Check sheet for the modelled part. Datum: model origin and axes. Units: mm. A direction names the side the tool comes from. Give positions to 0.01 mm unless a question says otherwise; leave off trailing zeros. Order: outer loops, then holes, each group sorted by start corner. A loop starts at its lowest first (then second) coordinate and runs counter-clockwise, first axis right, second up.
from build123d import *

# Parameters (mm, degrees)
F1_DEPTH  = 15
F3_DEPTH  = 2.6
F5_DEPTH  = 2.6
F6_R      = 2.5
F7_DEPTH  = 15.001
F9_DEPTH  = 25
F10_W     = 7.263658
F10_H     = 12.422406
F11_DEPTH = 25.43
F13_DEPTH = 13.301


with BuildPart() as f1:
    # F0 (on Top) → F1 (new body)
    with BuildSketch(Plane.XY):
        with BuildLine():
            Line((0, 10.7), (0, 0))
            Line((0, 0), (16.8, 0))
            Line((16.8, 0), (16.8, -2.6))
            Line((16.8, -2.6), (68.5, -2.6))
            Line((68.5, -2.6), (68.5, 3.1))
            Line((68.5, 3.1), (57, 3.1))
            ThreePointArc((57, 3.1), (54.75, 5.35), (57, 7.6))
            Line((57, 7.6), (68.5, 7.6))
            Line((68.5, 7.6), (68.5, 13.3))
            Line((68.5, 13.3), (16.8, 13.3))
            Line((16.8, 13.3), (16.8, 10.7))
            Line((16.8, 10.7), (0, 10.7))
        make_face()
        with BuildLine():
            Line((50.53, 0.57), (50.53, -1.1))
            Line((50.53, -1.1), (47.93, -1.1))
            Line((47.93, -1.1), (47.93, 0.37))
            Line((47.93, 0.37), (42.93, 0.37))
            Line((42.93, 0.37), (42.93, -1.1))
            Line((42.93, -1.1), (36.03, -1.1))
            Line((36.03, -1.1), (36.03, 11.8))
            Line((36.03, 11.8), (42.93, 11.8))
            Line((42.93, 11.8), (42.93, 10.33))
            Line((42.93, 10.33), (47.93, 10.33))
            Line((47.93, 10.33), (47.93, 11.8))
            Line((47.93, 11.8), (50.53, 11.8))
            Line((50.53, 11.8), (50.53, 10.13))
            ThreePointArc((50.53, 10.13), (45.75, 5.35), (50.53, 0.57))
        make_face(mode=Mode.SUBTRACT)
        with BuildLine():
            Line((25.897848, 2.656896), (25.897848, 0.656896))
            Line((25.897848, 0.656896), (24.897848, 0.656896))
            Line((24.897848, 0.656896), (23.134171, 1.6))
            Line((23.134171, 1.6), (10.6, 1.6))
            Line((10.6, 1.6), (10.6, 9.1))
            Line((10.6, 9.1), (23.134171, 9.1))
            Line((23.134171, 9.1), (24.897848, 10.043104))
            Line((24.897848, 10.043104), (25.897848, 10.043104))
            Line((25.897848, 10.043104), (25.897848, 8.043104))
            ThreePointArc((25.897848, 8.043104), (24.4, 5.35), (25.897848, 2.656896))
        make_face(mode=Mode.SUBTRACT)
    extrude(amount=F1_DEPTH)

    # F2 (on face) → F3 (cut, through all)
    with BuildSketch(Plane.XZ.offset(2.6)):
        Polygon((16.8, 15), (16.8, 0), (25.530007, 15), align=None)
    extrude(amount=-F3_DEPTH, mode=Mode.SUBTRACT)

    # F4 (on face) → F5 (cut, through all)
    with BuildSketch(Plane(origin=(0, 13.3, 0), x_dir=(-1, 0, 0), z_dir=(0, 1, 0))):
        Polygon((-25.53, 15), (-16.8, 0), (-16.8, 15), align=None)
    extrude(amount=-F5_DEPTH, mode=Mode.SUBTRACT)

    # F6 (on face) → F7 (cut, through all)
    with BuildSketch(Plane.XY.offset(15)):
        with Locations((30.779256, 5.35)):
            Circle(F6_R)
    extrude(amount=-F7_DEPTH, mode=Mode.SUBTRACT)

    # F8 (on face) → F9 (cut)
    with BuildSketch(Plane.YZ.offset(68.5)):
        Polygon((0, 13.7), (0, 0), (3.1, 0), (3.1, 9.610246), (1.181896, 10.552361), (1.181896, 13.7), align=None)
    extrude(amount=-F9_DEPTH, mode=Mode.SUBTRACT)

    # F10 (on face) → F11 (cut, through all)
    with BuildSketch(Plane.YZ.offset(36.03)):
        with Locations((5.951841, 7.195009)):
            Rectangle(F10_W, F10_H)
    extrude(amount=-F11_DEPTH, mode=Mode.SUBTRACT)

    # F12 (on face) → F13 (cut, through all)
    with BuildSketch(Plane.XZ):
        with BuildLine():
            ThreePointArc((0, 7.5), (1.970314, 9.507508), (4.698562, 8.822753))
            Line((4.698562, 8.822753), (25.530007, 15))
            Line((25.530007, 15), (0, 15))
            Line((0, 15), (0, 7.5))
        make_face()
    extrude(amount=-F13_DEPTH, mode=Mode.SUBTRACT)


solid = f1.part
1) Depth check by flat-ended pin: pin 1 Ø4 at (x, y) = (25.5, 4.5) entering from -Z; pin 2 Ø4 at (y, z) = (4, 6) entering from +X; pin 3 Ø6 at (x, z) = (14.5, 8.5) entering from -Y; pin 4 Ø2 at (x, z) = (8.5, 11.5) entering from +Y. Enter the tip coordinate at first touch or a pass-through.
Recorded:
pin 1: stops at z = 0
pin 2: stops at x = 57
pin 3: stops at y = 0
pin 4: passes through
2) Set-up check for faces 1 (the face through (10.436, 5.141, 10.524)), 2 (the face through (45, 10.33, 7)), 3 (the face through (57.562, 2.154, 10.075)), 4 (the face through (10, 10.7, 6)), 5 (the face through (63, 3.1, 12)): record each of +Z, -Z, +X, -X, +Y, -Y from which the full face is reachable in a straight line by a thin tool's end or side.
Recorded:
face 1: +Z, +Y, -Y
face 2: +Z, -Z
face 3: -Z, +X
face 4: +Z, -X, +Y
face 5: +Z, -Z, +X
3) Section check A-A, the plane x = 59.5. Record the cut outline in (y, z), then the cut area to 3 significant figures.
Recorded:
outline: (-2.6, 0) - (0, 0) - (0, 13.7) - (1.18, 13.7) - (1.18, 10.55) - (3.1, 9.61) - (3.1, 15) - (-2.6, 15) - close; (7.6, 0) - (13.3, 0) - (13.3, 15) - (7.6, 15) - close
area: 135 mm2
4) Material ranges on L1, parallel to Z at x = 26.5, y = 8.5; L2, parallel to Y at x = 65.5, z = 8; L3, parallel to X at y = 5.5, z = 2.5 (3 decimals), recorded low to high.
Recorded:
L1: z = 0 to 0.98, 13.41 to 15
L2: y = -2.6 to 0, 7.6 to 13.3
L3: x = 0 to 10.6, 45.752 to 54.755
5) Section check B-B, the plane y = 5.35. Record the cut outline in (x, z), then the cut area to 3 significant figures.
Recorded:
outline: (0, 0) - (10.6, 0) - (10.6, 10.57) - (4.7, 8.82) arc R2.83 ccw to (0, 7.5) - close; (24.4, 0) - (28.28, 0) - (28.28, 0.98) - (24.4, 0.98) - close; (24.4, 13.41) - (28.28, 13.41) - (28.28, 15) - (25.53, 15) - (24.4, 14.66) - close; (33.28, 0) - (36.03, 0) - (36.03, 0.98) - (33.28, 0.98) - close; (33.28, 13.41) - (36.03, 13.41) - (36.03, 15) - (33.28, 15) - close; (45.75, 0) - (54.75, 0) - (54.75, 15) - (45.75, 15) - close
area: 252 mm2
6) Section check C-C, the plane x = 19. Record the cut outline in (y, z), then the cut area to 3 significant figures.
Recorded:
outline: (-2.6, 0) - (1.6, 0) - (1.6, 13.06) - (0, 13.06) - (0, 3.78) - (-2.6, 3.78) - close; (9.1, 0) - (13.3, 0) - (13.3, 3.78) - (10.7, 3.78) - (10.7, 13.06) - (9.58, 13.06) - (9.58, 0.98) - (9.1, 0.98) - close
area: 55.6 mm2
7) Section check D-D, the plane x = 31.5. Record the cut outline in (y, z).
Recorded:
outline: (-2.6, 0) - (2.96, 0) - (2.96, 0.98) - (2.32, 0.98) - (2.32, 13.41) - (2.96, 13.41) - (2.96, 15) - (-2.6, 15) - close; (7.74, 0) - (13.3, 0) - (13.3, 15) - (7.74, 15) - (7.74, 13.41) - (9.58, 13.41) - (9.58, 0.98) - (7.74, 0.98) - close
8) Draft check along Y on faces 6 (the face through (13, 0, 6)), 7 (the face through (68.5, 10, 7)), 8 (the face through (52, 3.1, 5)), 9 (the face through (28.28, 5.46, 0.5)). Enter one of: +Y half, -Y half, draft (parallel to the pull), parting line (faces both ways), or undercut.
Recorded:
face 6: -Y half
face 7: draft
face 8: undercut
face 9: undercut
